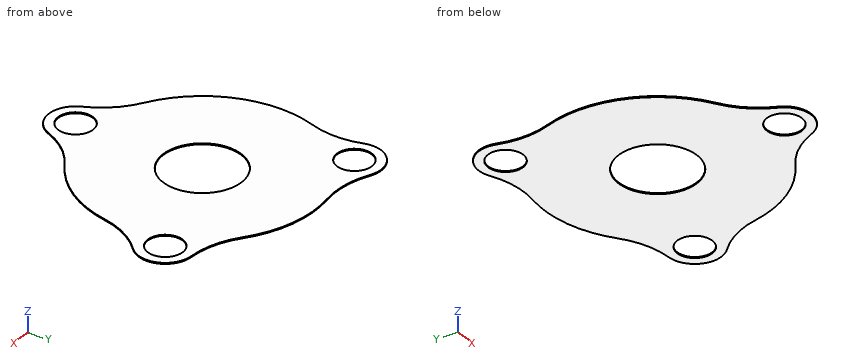
from build123d import *

# Parameters (mm, degrees)
SKETCH1_R      = 8.5
SKETCH1_R_2    = 19
EXTRUDE1_DEPTH = 0.5


with BuildPart() as part:
    # Sketch1 → Extrude1 (new body)
    with BuildSketch(Plane.XY):
        with BuildLine():
            ThreePointArc((-11.993220936, -66.016238788), (0, -74), (11.993220936, -66.016238788))
            ThreePointArc((11.993220936, -66.016238788), (18.643198205, -55.282099515), (28.307885854, -47.155737705))
            ThreePointArc((28.307885854, -47.155737705), (45.053362436, -31.546703999), (53.993765926, -10.472499278))
            ThreePointArc((53.993765926, -10.472499278), (58.324530298, 1.388715818), (66.136895584, 11.308942239))
            ThreePointArc((66.136895584, 11.308942239), (69.537253938, 25.309490606), (57.933049297, 33.848824665))
            ThreePointArc((57.933049297, 33.848824665), (45.571831653, 36.426467381), (34.630031572, 42.728923615))
            ThreePointArc((34.630031572, 42.728923615), (14.235047481, 53.125920446), (-8.626025268, 54.319349113))
            ThreePointArc((-8.626025268, 54.319349113), (-21.253130218, 54.332161948), (-33.247080077, 58.280466697))
            ThreePointArc((-33.247080077, 58.280466697), (-47.566283117, 56.687288791), (-51.621760584, 42.862279061))
            ThreePointArc((-51.621760584, 42.862279061), (-49.816166993, 30.364928326), (-51.996222577, 17.927432547))
            ThreePointArc((-51.996222577, 17.927432547), (-51.683094143, -18.811107883), (-28.307885854, -47.155737705))
            ThreePointArc((-28.307885854, -47.155737705), (-18.643198205, -55.282099515), (-11.993220936, -66.016238788))
        make_face()
        with Locations((57.321249868, 20.863228743)):
            Circle(SKETCH1_R, mode=Mode.SUBTRACT)
        with Locations((-39.210044191, 46.72871103)):
            Circle(SKETCH1_R, mode=Mode.SUBTRACT)
        with Locations((0, -61)):
            Circle(SKETCH1_R, mode=Mode.SUBTRACT)
        Circle(SKETCH1_R_2, mode=Mode.SUBTRACT)
    extrude(amount=EXTRUDE1_DEPTH)


solid = part.part
Geometry check sheet. Reference: the model listing, model coordinates, mm. Round coordinates to 2 decimals unless told otherwise and drop trailing zeros. Loops run counter-clockwise (first coordinate to the right, second up) from the corner with the lowest first, then second, coordinate; pieces in that order, holes last. Notation, with made-up numbers: (13, 18) - (29, 18) arc R15 cw to (29, 31) - close; hole circle Ø6 at (49, 70.25). An arc over 180 degrees is marked (long way). Answer as CSV lines item,"result".
(1) Cross-section at A-A, the plane x = 0. Enter the section's corners in (y, z), and give its area (3 significant figures).
Output values:
outline,"(-74, 0) - (-69.5, 0) - (-69.5, 0.5) - (-74, 0.5) - close; (-52.5, 0) - (-19, 0) - (-19, 0.5) - (-52.5, 0.5) - close; (19, 0) - (55, 0) - (55, 0.5) - (19, 0.5) - close"
area,"37.0 mm²"
(2) Material ranges on line 1 along Y through (x, z) = (0, 0.3); line 2 along X through (y, z) = (13, 0.15); line 3 along Y through (x, z) = (-13.5, 0.1), recorded low to high.
Output values:
line 1,"y = -74 to -69.5, -52.5 to -19, 19 to 55"
line 2,"x = -53.44 to -13.86, 13.86 to 54.09, 60.55 to 67.67"
line 3,"y = -62.82 to -13.37, 13.37 to 53.85"
(3) Cross-section at B-B, the plane y = 0. Enter the section's corners in (x, z).
Output values:
outline,"(-55, 0) - (-19, 0) - (-19, 0.5) - (-55, 0.5) - close; (19, 0) - (57.59, 0) - (57.59, 0.5) - (19, 0.5) - close"
(4) Cross-section at C-C, the plane z = 0.3. Enter the section's corners in (x, y), and give its area (3 significant figures).
Output values:
outline,"(-52, 17.93) arc R55 ccw to (-28.31, -47.16) arc R40 cw to (-11.99, -66.02) arc R13 ccw to (11.99, -66.02) arc R40 cw to (28.31, -47.16) arc R55 ccw to (53.99, -10.47) arc R40 cw to (66.14, 11.31) arc R13 ccw to (57.93, 33.85) arc R40 cw to (34.63, 42.73) arc R55 ccw to (-8.63, 54.32) arc R40 cw to (-33.25, 58.28) arc R13 ccw to (-51.62, 42.86) arc R40 cw to start; hole circle Ø17 at (-39.21, 46.73); hole circle Ø38 at (0, 0); hole circle Ø17 at (0, -61); hole circle Ø17 at (57.32, 20.86)"
area,"9,280 mm²"
(5) Cross-section at D-D, the plane y = -61. Enter the section's corners in (x, z).
Output values:
outline,"(-14.52, 0) - (-8.5, 0) - (-8.5, 0.5) - (-14.52, 0.5) - close; (8.5, 0) - (14.52, 0) - (14.52, 0.5) - (8.5, 0.5) - close"
